Work out the finished part from the listing and answer in its coordinate system (mm). Face numbers are marked on the shaded views. A direction names the side the tool comes from. Coordinates: 2 decimals unless noted, no trailing zeros. Write each loop counter-clockwise with the first axis right and the second up, starting at its lowest first coordinate (ties: lowest second). Pieces come first, ordered by that corner, then holes. Notation, with made-up numbers: M 76,74.5 L 110,74.5 A20 ccw 110,103.5 Z; hole C -2.75,33 d2. An arc over 180 degrees is marked long. Use CSV: the item, a comma, the result in double quotes.
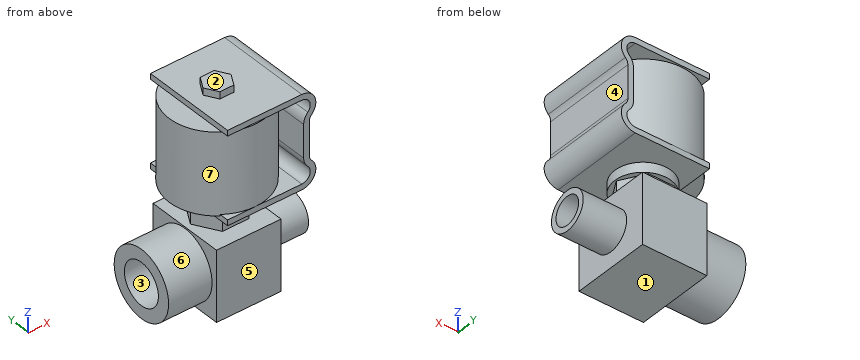
from build123d import *

# Parameters (mm, degrees)
PAD004_DEPTH            = 34
CYLINDER001_R           = 5
CYLINDER001_DEPTH       = 16
CYLINDER001_PITCH_ANGLE = 90
CYLINDER003_R           = 7
CYLINDER003_DEPTH       = 16
CYLINDER003_PITCH_ANGLE = 90
CYLINDER002_R           = 7.5
CYLINDER002_DEPTH       = 16
CYLINDER002_PITCH_ANGLE = 90
CYLINDER_R              = 12
CYLINDER_DEPTH          = 16
CYLINDER_PITCH_ANGLE    = 90
BOX_W                   = 23
BOX_H                   = 28
BOX_DEPTH               = 25
PAD_DEPTH               = 6
SKETCH001_R             = 10
PAD001_DEPTH            = 5
SKETCH002_R             = 17
PAD002_DEPTH            = 29
PAD003_DEPTH            = 5


with BuildPart() as pad004:
    # Sketch004 → Pad004 (new body)
    with BuildSketch(Plane.XZ.offset(-17)):
        with BuildLine():
            Line((-10, 55), (16.5, 55))
            ThreePointArc((20.035534, 46.464466), (21.119398, 51.913417), (16.5, 55))
            ThreePointArc((20.035534, 46.464466), (19.385216, 45.491196), (19.156854, 44.343146))
            Line((19.156854, 44.343146), (19.156854, 32.656854))
            ThreePointArc((19.156854, 32.656854), (19.384362, 31.50845), (20.035534, 30.535534))
            ThreePointArc((16.5, 22), (21.119398, 25.086583), (20.035534, 30.535534))
            Line((-10, 22), (16.5, 22))
            Line((-10, 24), (-10, 22))
            Line((-10, 24), (16.5, 24))
            ThreePointArc((16.5, 24), (19.271639, 25.85195), (18.62132, 29.12132))
            ThreePointArc((17.156854, 32.656854), (17.537457, 30.743437), (18.62132, 29.12132))
            Line((17.156854, 44.343146), (17.156854, 32.656854))
            ThreePointArc((18.62132, 47.87868), (17.537457, 46.256563), (17.156854, 44.343146))
            ThreePointArc((18.62132, 47.87868), (19.271639, 51.14805), (16.5, 53))
            Line((-10, 53), (16.5, 53))
            Line((-10, 55), (-10, 53))
        make_face()
    extrude(amount=PAD004_DEPTH)


with BuildPart() as cylinder001:
    # Cylinder001 → Cylinder001 (new body)
    with BuildSketch(Plane.XY):
        Circle(CYLINDER001_R)
    extrude(amount=CYLINDER001_DEPTH)


with BuildPart() as cylinder001_1:
    # Cylinder001 pitch: moved
    add(cylinder001.part.rotate(Axis((0, 0, 0), (0, 1, 0)), CYLINDER001_PITCH_ANGLE))


with BuildPart() as cylinder001_2:
    # Cylinder001 placement: moved
    add(cylinder001_1.part.moved(Location((11, 0, 0))))


with BuildPart() as cut001:
    # Cylinder003 → Cylinder003 (new body)
    with BuildSketch(Plane.XY):
        Circle(CYLINDER003_R)
    extrude(amount=CYLINDER003_DEPTH)


with BuildPart() as cut001_1:
    # Cylinder003 pitch: moved
    add(cut001.part.rotate(Axis((0, 0, 0), (0, 1, 0)), CYLINDER003_PITCH_ANGLE))


with BuildPart() as cut001_2:
    # Cylinder003 placement: moved
    add(cut001_1.part.moved(Location((11, 0, 0))))

    # Cut001: cut Cylinder001
    add(cylinder001_2.part, mode=Mode.SUBTRACT)


with BuildPart() as cylinder002:
    # Cylinder002 → Cylinder002 (new body)
    with BuildSketch(Plane.XY):
        Circle(CYLINDER002_R)
    extrude(amount=CYLINDER002_DEPTH)


with BuildPart() as cylinder002_1:
    # Cylinder002 pitch: moved
    add(cylinder002.part.rotate(Axis((0, 0, 0), (0, 1, 0)), CYLINDER002_PITCH_ANGLE))


with BuildPart() as cylinder002_2:
    # Cylinder002 placement: moved
    add(cylinder002_1.part.moved(Location((-27, 0, 0))))


with BuildPart() as cut:
    # Cylinder → Cylinder (new body)
    with BuildSketch(Plane.XY):
        Circle(CYLINDER_R)
    extrude(amount=CYLINDER_DEPTH)


with BuildPart() as cut_1:
    # Cylinder pitch: moved
    add(cut.part.rotate(Axis((0, 0, 0), (0, 1, 0)), CYLINDER_PITCH_ANGLE))


with BuildPart() as cut_2:
    # Cylinder placement: moved
    add(cut_1.part.moved(Location((-27, 0, 0))))

    # Cut: cut Cylinder002
    add(cylinder002_2.part, mode=Mode.SUBTRACT)


with BuildPart() as fusion002:
    # Box → Box (new body)
    with BuildSketch(Plane(origin=(-11.5, -14, -12.5), x_dir=(1, 0, 0), z_dir=(0, 0, 1))):
        with Locations((11.5, 14)):
            Rectangle(BOX_W, BOX_H)
    extrude(amount=BOX_DEPTH)

    # Fusion: union Cut
    add(cut_2.part)

    # Fusion001: union Cut001
    add(cut001_2.part)

    # Sketch → Pad (new body)
    with BuildSketch(Plane.XY.offset(12.5)):
        Polygon((4.75, 8.227241), (-4.75, 8.227241), (-9.5, 0), (-4.75, -8.227241), (4.75, -8.227241), (9.5, 0), align=None)
    extrude(amount=PAD_DEPTH)

    # Sketch001 → Pad001 (new body)
    with BuildSketch(Plane.XY.offset(18.5)):
        Circle(SKETCH001_R)
    extrude(amount=PAD001_DEPTH)

    # Sketch002 → Pad002 (new body)
    with BuildSketch(Plane.XY.offset(23.5)):
        Circle(SKETCH002_R)
    extrude(amount=PAD002_DEPTH)

    # Sketch003 → Pad003 (new body)
    with BuildSketch(Plane.XY.offset(52.5)):
        Polygon((2.5, 4.330127), (-2.5, 4.330127), (-5, 0), (-2.5, -4.330127), (2.5, -4.330127), (5, 0), align=None)
    extrude(amount=PAD003_DEPTH)

    # Fusion002: union Pad004
    add(pad004.part)


solid = fusion002.part
Item 1: For a pull along Z with two mould halves and no side action, classify the marked faces 1, 2 and 3 as released by +Z, released by -Z, zero draft, split by the parting line, or undercut.
Answer:
face 1,"released by -Z"
face 2,"released by +Z"
face 3,"undercut"
Item 2: The part is cut by section B-B (x = -13). Write down the section's boundary in (y, z).
Answer:
outline,"C 0,0 d24; M -10.95,23.5 L 10.95,23.5 L 10.95,52.5 L -10.95,52.5 Z; hole C 0,0 d15"
Item 3: The part is cut by section A-A (z = 41). Write down the section's boundary in (x, y).
Answer:
outline,"C 0,0 d34; M 17.16,-17 L 19.16,-17 L 19.16,17 L 17.16,17 Z"
Item 4: Given pin 1 (1 mm diameter, centred on y = 0.5, z = 34, fed in from +X); pin 2 (3.5 mm diameter, centred on y = -2.5, z = 36, fed in from -X); pin 3 (4 mm diameter, centred on x = -4.5, z = 16, fed in from -Y), each flat-ended and moving along its own axis, determine where each tip first touches the part or whether it passes through.
Answer:
pin 1,"stops at x = 19.16"
pin 2,"stops at x = -16.98"
pin 3,"stops at y = -8.23"
Item 5: A tool of negligible diameter and unlimited length cuts with its end or side. For the marked faces 4, 5, 6 and 7, from which of +Z, -Z, +X, -X, +Y, -Y can it reach the whole face along a straight path? Write none if from no direction.
Answer:
face 4,"+X, +Y, -Y"
face 5,"-Z, +X, -X, -Y"
face 6,"-X"
face 7,"none"
Item 6: Consider probe 1 along Z at (x, y) = (-15.75, 0); probe 2 along Z at (x, y) = (4, 8.5); probe 3 along Y at (x, z) = (-23, 0). Determine where each line is inside the solid, lowest interval first.
Answer:
probe 1,"z = -12 to -7.5, 7.5 to 12, 23.5 to 52.5"
probe 2,"z = -12.5 to 12.5, 18.5 to 52.5, 53 to 55"
probe 3,"y = -12 to -7.5, 7.5 to 12"
Item 7: The part is cut by section C-C (y = 15). Write down the section's boundary in (x, z).
Answer:
outline,"M -10,22 L 16.5,22 A5 ccw 20.04,30.54 A2.99 cw 19.16,32.66 L 19.16,44.34 A3 cw 20.04,46.46 A5 ccw 16.5,55 L -10,55 L -10,53 L 16.5,53 A3 cw 18.62,47.88 A5 ccw 17.16,44.34 L 17.16,32.66 A5 ccw 18.62,29.12 A3 cw 16.5,24 L 8,24 L 8,52.5 L -8,52.5 L -8,24 L -10,24 Z"
Item 8: The part is cut by section D-D (z = 0). Write down the section's boundary in (x, y), then the cut area to 4 significant figures.
Answer:
outline,"M -27,-12 L -11.5,-12 L -11.5,-14 L 11.5,-14 L 11.5,-7 L 27,-7 L 27,-5 L 11.5,-5 L 11.5,5 L 27,5 L 27,7 L 11.5,7 L 11.5,14 L -11.5,14 L -11.5,12 L -27,12 L -27,7.5 L -11.5,7.5 L -11.5,-7.5 L -27,-7.5 Z"
area,"845.5 mm2"
